Input: part model. Units: mm. Frame: model coordinates. Face numbers are marked on the shaded views. Coordinates: 2 decimals unless noted, no trailing zeros. Write each loop counter-clockwise with the first axis right and the second up, starting at its lowest first coordinate (ties: lowest second). Pieces come first, ordered by that corner, then holes. Notation, with made-up numbers: M -19,-15 L 40,-15 A5 ccw 40,-10 Z; hole C -13.75,-36.75 d5. An arc over 180 degrees is marked long. Write each question's results on one line, items separated by ' | '. Start each with the question number.
1. Section query B-B, the plane z = -326. Output: boundary loops of the cut face in (x, y).
2. First-contact query: pin 1 (12 mm diameter, centred on x = 261.5, y = -481.5, fed in from +Z). Flat tip, straight axial feed; report the tip coordinate or a pass-through.
3. Pull-direction query (X, two-part tool) for the marked faces 1 and 2; classes: +X half, -X half, draft (parallel to the pull), parting line (faces both ways), or undercut.
4. Ray query, probe 1 along Z at (x, y) = (28, -270); probe 2 along X at (y, z) = (-203, -23); probe 3 along Y at (x, z) = (158, -56). Return the intervals inside material, ascending.
5. Section query C-C, the plane x = 66.5. Output: boundary loops of the cut face in (y, z).
6. Section query A-A, the plane y = -222. Output: boundary loops of the cut face in (x, z), and give its area (3 significant figures).
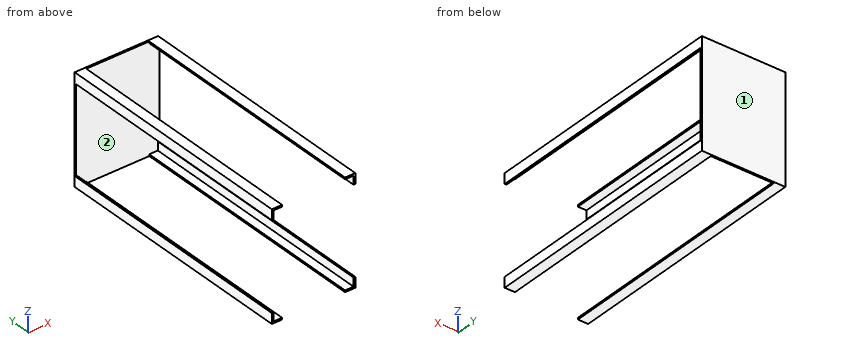
```python
from build123d import *

# Parameters (mm, degrees)
CROQUIS2_W              = 310
CROQUIS2_H              = 400
SALIENTE_EXTRUIR1_DEPTH = 6.35
SALIENTE_EXTRUIR2_DEPTH = 920


with BuildPart() as part:
    # Croquis2 → Saliente-Extruir1 (new body)
    with BuildSketch(Plane(origin=(0, 0, 0), x_dir=(1, 0, 0), z_dir=(0, 1, 0))):
        with Locations((155, 200)):
            Rectangle(CROQUIS2_W, CROQUIS2_H)
    extrude(amount=-SALIENTE_EXTRUIR1_DEPTH)

    # Croquis3 → Saliente-Extruir2 (add)
    with BuildSketch(Plane.XZ.offset(6.35)):
        Polygon((0, 0), (38.1, 0), (38.1, -6.35), (6.35, -6.35), (6.35, -38.1), (0, -38.1), align=None)
        Polygon((303.65, -38.1), (310, -38.1), (310, 0), (271.9, 0), (271.9, -6.35), (303.65, -6.35), align=None)
        Polygon((310, -400), (271.9, -400), (271.9, -393.65), (303.65, -393.65), (303.65, -361.9), (310, -361.9), align=None)
        Polygon((6.35, -361.9), (0, -361.9), (0, -400), (38.1, -400), (38.1, -393.65), (6.35, -393.65), align=None)
    extrude(amount=SALIENTE_EXTRUIR2_DEPTH)


solid = part.part
```
Answer:
1) outline: M 0,-6.35 L 310,-6.35 L 310,0 L 0,0 Z
2) pin 1: through
3) face 1: draft | face 2: undercut
4) probe 1: -400 to -393.65, -6.35 to 0 | probe 2: 0 to 6.35, 303.65 to 310 | probe 3: -6.35 to 0
5) outline: M -6.35,-400 L 0,-400 L 0,0 L -6.35,0 Z
6) outline: M 0,-400 L 38.1,-400 L 38.1,-393.65 L 6.35,-393.65 L 6.35,-361.9 L 0,-361.9 Z; M 0,-38.1 L 6.35,-38.1 L 6.35,-6.35 L 38.1,-6.35 L 38.1,0 L 0,0 Z; M 271.9,-400 L 310,-400 L 310,-361.9 L 303.65,-361.9 L 303.65,-393.65 L 271.9,-393.65 Z; M 271.9,-6.35 L 303.65,-6.35 L 303.65,-38.1 L 310,-38.1 L 310,0 L 271.9,0 Z | area: 1,770 mm^2
